Design review of the part built by this model. Coordinates are the model's own, in mm. Round coordinates to 2 decimals unless told otherwise and drop trailing zeros. Order: outer loops, then holes, each group sorted by start corner. A loop starts at its lowest first (then second) coordinate and runs counter-clockwise, first axis right, second up. Notation, with made-up numbers: (23, 53) - (52, 53) arc R18 cw to (52, 80) - close; hole circle Ø10 at (41.5, 58). An arc over 180 degrees is marked (long way). Use CSV: the item, a comma, the result in double quotes.
from build123d import *

# Parameters (mm, degrees)
F0_R     = 50.1004496622
F1_DEPTH = 12.7
F2_SIZE  = 6.35
F3_SIZE  = 6.34999


# Not quite as in the source:
# - a fillet or chamfer is up to 0.001 mm smaller than in the source, because OpenCascade refuses the exact size


with BuildPart() as f1:
    # F0 (on Top) → F1 (new body)
    with BuildSketch(Plane.XY):
        with Locations((-3.3122645349, -2.7786610853)):
            Circle(F0_R)
    extrude(amount=F1_DEPTH)

    # F2
    f2_edges = [f1.edges().sort_by_distance(p)[0] for p in [
        (-53.412714, -2.778661, 12.7),
    ]]
    chamfer(f2_edges, length=F2_SIZE)

    # F3 (size 6.35 in the source; OpenCascade refuses exactly that, so slightly less here)
    f3_edges = [f1.edges().sort_by_distance(p)[0] for p in [
        (-53.412714, -2.778661, 0),
    ]]
    chamfer(f3_edges, length=F3_SIZE)


solid = f1.part
1) To check wall thickness, follow L1, parallel to X at y = -9, z = 3.75; L2, parallel to Y at x = -3.5, z = 9; L3, parallel to Y at x = -26, z = 3. State the ranges of each line that lie inside material, in increasing order. Write a range as from..to.
Data:
L1,"x = -50.4..43.78"
L2,"y = -50.23..44.67"
L3,"y = -43.65..38.1"
2) Insertion check: pin 1 Ø4 at (x, z) = (-22.5, 2) entering from -Y; pin 2 Ø3 at (x, z) = (-27, 8) entering from +Y; pin 3 Ø2 at (y, z) = (-7, 3.5) entering from -X. Each pin has a flat end and moves straight along its axis. Give the tip position at first contact, or say it passes through.
Data:
pin 1,"stops at y = -46.67"
pin 2,"stops at y = 41.38"
pin 3,"stops at x = -51.38"
3) We need section A-A (z = 10.5). Give the boundary of the cut face in (x, y).
Data:
outline,"circle Ø91.9 at (-3.31, -2.78)"
4) We need section B-B (z = 3.25). Give the boundary of the cut face in (x, y).
Data:
outline,"circle Ø94 at (-3.31, -2.78)"
